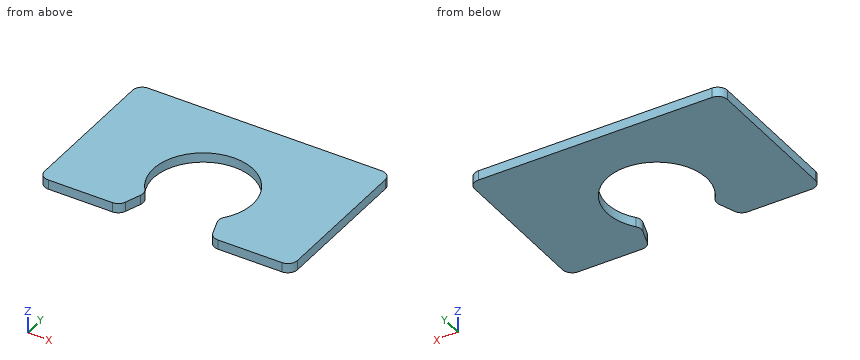
```python
from build123d import *

# Parameters (mm, degrees)
F1_DEPTH    = 25
F2_T1_DEPTH = 150
F2_T3_DEPTH = 113.556925296
F2_T5_DEPTH = 96.327528549
F2_T7_DEPTH = 96.2047902339
F2_T9_DEPTH = 113.6738307778


# Not quite as in the source:
# - a fillet or chamfer that OpenCascade refuses, or shapes differently, is made with other operations: its cross-section is extruded or revolved along the edge and cut away or added


with BuildPart() as f1:
    # F0 (on Top) → F1 (new body)
    with BuildSketch(Plane.XY):
        with BuildLine():
            Line((330, -210), (330, 210))
            Line((330, 210), (-330, 210))
            Line((-330, 210), (-330, -210))
            Line((-330, -210), (-120, -210))
            Line((-120, -210), (-94.9556464673, -138.7567549117))
            ThreePointArc((-94.9556464673, -138.7567549117), (-47.6770453611, 70.9299598508), (130.0298179868, -50))
            ThreePointArc((130.0298179868, -50), (120.9675904588, -97.6870547372), (95.0443535327, -138.7256334719))
            Line((95.0443535327, -138.7256334719), (120, -210))
            Line((120, -210), (330, -210))
        make_face()
    extrude(amount=F1_DEPTH)

    # F2: fillet of radius 25 on 9 edges, made by hand

    # F2_s2 → F2_t1 (cut)
    with BuildSketch(Plane.XY.offset(-62.5)):
        with BuildLine():
            ThreePointArc((330, -185), (322.6776695297, -202.6776695297), (305, -210))
            Line((305, -210), (330, -210))
            Line((330, -210), (330, -185))
        make_face()
        with BuildLine():
            ThreePointArc((-330, -185), (-322.6776695297, -202.6776695297), (-305, -210))
            Line((-305, -210), (-330, -210))
            Line((-330, -210), (-330, -185))
        make_face()
        with BuildLine():
            ThreePointArc((330, 185), (322.6776695297, 202.6776695297), (305, 210))
            Line((305, 210), (330, 210))
            Line((330, 210), (330, 185))
        make_face()
        with BuildLine():
            ThreePointArc((-305, 210), (-322.6776695297, 202.6776695297), (-330, 185))
            Line((-330, 185), (-330, 210))
            Line((-330, 210), (-305, 210))
        make_face()
    extrude(amount=F2_T1_DEPTH, mode=Mode.SUBTRACT)

    # F2_s4 → F2_t3 (cut)
    with BuildSketch(Plane.XY.offset(-44.278462648)):
        with BuildLine():
            ThreePointArc((-137.7113850592, -210), (-123.2592934135, -205.3994374203), (-114.1262219297, -193.2909637652))
            Line((-114.1262219297, -193.2909637652), (-120, -210))
            Line((-120, -210), (-137.7113850592, -210))
        make_face()
    extrude(amount=F2_T3_DEPTH, mode=Mode.SUBTRACT)

    # F2_s6 → F2_t5 (cut)
    with BuildSketch(Plane.XY.offset(-35.6637642745)):
        with BuildLine():
            ThreePointArc((-99.6866381045, -152.2149260833), (-98.5772005252, -140.0282344234), (-103.3844432952, -128.7749361378))
            ThreePointArc((-103.3844432952, -128.7749361378), (-99.2955159897, -133.8717952023), (-94.9556464673, -138.7567549117))
            Line((-94.9556464673, -138.7567549117), (-99.6866381045, -152.2149260833))
        make_face()
    extrude(amount=F2_T5_DEPTH, mode=Mode.SUBTRACT)

    # F2_s8 → F2_t7 (cut)
    with BuildSketch(Plane.XY.offset(-35.6023951169)):
        with BuildLine():
            ThreePointArc((103.4562444176, -128.7589633994), (98.6534687448, -139.9957269325), (99.7504758881, -152.1665150823))
            Line((99.7504758881, -152.1665150823), (95.0443535327, -138.7256334719))
            ThreePointArc((95.0443535327, -138.7256334719), (99.3753638137, -133.8478534272), (103.4562444176, -128.7589633994))
        make_face()
    extrude(amount=F2_T7_DEPTH, mode=Mode.SUBTRACT)

    # F2_s10 → F2_t9 (cut)
    with BuildSketch(Plane.XY.offset(-44.3369153889)):
        with BuildLine():
            ThreePointArc((114.1393002355, -193.261597183), (123.2699801146, -205.3904380725), (137.7347661556, -210))
            Line((137.7347661556, -210), (120, -210))
            Line((120, -210), (114.1393002355, -193.261597183))
        make_face()
    extrude(amount=F2_T9_DEPTH, mode=Mode.SUBTRACT)


solid = f1.part
```
The listing builds one solid part. Answer for the finished solid, in the listing's coordinates (mm). Round coordinates to 2 decimals unless told otherwise and drop trailing zeros. Loops run counter-clockwise (first coordinate to the right, second up) from the corner with the lowest first, then second, coordinate; pieces in that order, holes last. Notation, with made-up numbers: (-7, 47.25) - (-3, 47.25) arc R28 cw to (-3, 77.25) - close; hole circle Ø9 at (52.5, -20.75). An arc over 180 degrees is marked (long way). Use one line per item in the form item = value. Start each with the question number.
1. The part is cut by section B-B on z = 19.75. Determine the outline of the cut face in (x, y).
2. The part is cut by section A-A on y = -50. Determine the outline of the cut face in (x, z).
3. Consider line 1 (X direction, y = -50, z = 7); line 2 (X direction, y = 52.5, z = 17.5); line 3 (Y direction, x = 36, z = 10.75). Determine where each line is inside the solid, lowest interval first. Write a range as [from, to].
Geometry check:
q1.outline = (-330, -185) arc R25 ccw to (-305, -210) - (-137.71, -210) arc R25 ccw to (-114.13, -193.29) - (-99.69, -152.21) arc R25 ccw to (-103.38, -128.77) arc R130 cw (long way) to (103.46, -128.76) arc R25 ccw to (99.75, -152.17) - (114.14, -193.26) arc R25 ccw to (137.73, -210) - (305, -210) arc R25 ccw to (330, -185) - (330, 185) arc R25 ccw to (305, 210) - (-305, 210) arc R25 ccw to (-330, 185) - close
q2.outline = (-330, 0) - (-129.97, 0) - (-129.97, 25) - (-330, 25) - close; (130.03, 0) - (330, 0) - (330, 25) - (130.03, 25) - close
q3.line_1 = [-330, -129.97], [130.03, 330]
q3.line_2 = [-330, -79.93], [79.99, 330]
q3.line_3 = [74.92, 210]
